Build history of the part. All positions in model axes, mm. Give positions to 0.01 mm unless a question says otherwise; leave off trailing zeros. Order: outer loops, then holes, each group sorted by start corner. A loop starts at its lowest first (then second) coordinate and runs counter-clockwise, first axis right, second up. Notation, with made-up numbers: (-15.75, -29.5) - (-4.75, -29.5) arc R22 ccw to (-4.75, -16.5) - close; hole circle Ø9 at (-6.5, 84.5). An arc over 180 degrees is marked (long way). Use a Markdown table: item, result.
from build123d import *

# Parameters (mm, degrees)
SKETCH2_W           = 30
SKETCH2_H           = 165
BOSS_EXTRUDE1_DEPTH = 8
SKETCH3_R           = 2.75
CUT_EXTRUDE1_DEPTH  = 8
SKETCH4_R           = 5
CUT_EXTRUDE2_DEPTH  = 4.2
SKETCH5_R           = 2.5
CUT_EXTRUDE3_DEPTH  = 41.2


with BuildPart() as part:
    # Sketch2 → Boss-Extrude1 (new body)
    with BuildSketch(Plane(origin=(0, 0, 0), x_dir=(1, 0, 0), z_dir=(0, 1, 0))):
        Rectangle(SKETCH2_W, SKETCH2_H)
    extrude(amount=BOSS_EXTRUDE1_DEPTH)

    # Sketch3 → Cut-Extrude1 (cut)
    with BuildSketch(Plane(origin=(0, 8, 0), x_dir=(1, 0, 0), z_dir=(0, 1, 0))):
        with Locations((0, -76.5)):
            Circle(SKETCH3_R)
        with Locations((0, 76.5)):
            Circle(SKETCH3_R)
    extrude(amount=-CUT_EXTRUDE1_DEPTH, mode=Mode.SUBTRACT)

    # Sketch4 → Cut-Extrude2 (cut)
    with BuildSketch(Plane(origin=(0, 8, 0), x_dir=(1, 0, 0), z_dir=(0, 1, 0))):
        with Locations((0, 76.5)):
            Circle(SKETCH4_R)
        with Locations((0, -76.5)):
            Circle(SKETCH4_R)
    extrude(amount=-CUT_EXTRUDE2_DEPTH, mode=Mode.SUBTRACT)

    # Sketch5 → Cut-Extrude3 (cut)
    with BuildSketch(Plane(origin=(0, 8, 0), x_dir=(1, 0, 0), z_dir=(0, 1, 0))):
        with Locations((-10, 76.5)):
            Circle(SKETCH5_R)
        with Locations((10, 76.5)):
            Circle(SKETCH5_R)
        with Locations((-10, -76.5)):
            Circle(SKETCH5_R)
        with Locations((10, -76.5)):
            Circle(SKETCH5_R)
    extrude(amount=-CUT_EXTRUDE3_DEPTH, mode=Mode.SUBTRACT)


solid = part.part
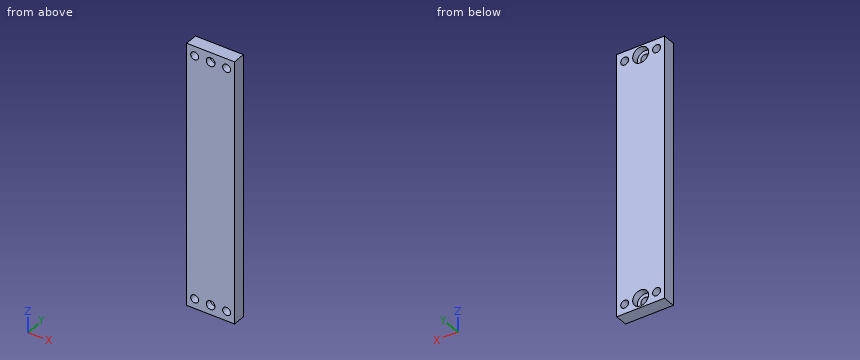
1) Wall check: line 1 (Z direction, x = 0, y = 5.6); line 2 (X direction, y = 3.5, z = 76.5); line 3 (Z direction, x = -10, y = 6.25). Give the ranges that are in metal, low to high. Write a range as from..to.
Computed:
| item | result |
|---|---|
| line 1 | z = -82.5..-81.5, -71.5..71.5, 81.5..82.5 |
| line 2 | x = -15..-12.5, -7.5..-2.75, 2.75..7.5, 12.5..15 |
| line 3 | z = -82.5..-79, -74..74, 79..82.5 |
2) Slice it at C-C (y = 6.5). Write the cut outline in (x, z), and give its area (3 significant figures).
Computed:
| item | result |
|---|---|
| outline | (-15, -82.5) - (15, -82.5) - (15, 82.5) - (-15, 82.5) - close; hole circle Ø5 at (-10, -76.5); hole circle Ø5 at (-10, 76.5); hole circle Ø10 at (0, -76.5); hole circle Ø10 at (0, 76.5); hole circle Ø5 at (10, -76.5); hole circle Ø5 at (10, 76.5) |
| area | 4,710 mm² |
3) Slice it at D-D (x = -10). Write the cut outline in (y, z).
Computed:
| item | result |
|---|---|
| outline | (0, -82.5) - (8, -82.5) - (8, -79) - (0, -79) - close; (0, -74) - (8, -74) - (8, 74) - (0, 74) - close; (0, 79) - (8, 79) - (8, 82.5) - (0, 82.5) - close |
4) Slice it at B-B (x = 0). Write the cut outline in (y, z), and give its area (3 significant figures).
Computed:
| item | result |
|---|---|
| outline | (0, -82.5) - (8, -82.5) - (8, -81.5) - (3.8, -81.5) - (3.8, -79.25) - (0, -79.25) - close; (0, -73.75) - (3.8, -73.75) - (3.8, -71.5) - (8, -71.5) - (8, 71.5) - (3.8, 71.5) - (3.8, 73.75) - (0, 73.75) - close; (0, 79.25) - (3.8, 79.25) - (3.8, 81.5) - (8, 81.5) - (8, 82.5) - (0, 82.5) - close |
| area | 1,190 mm² |
5) Slice it at A-A (z = -76.5). Write the cut outline in (x, y), and give its area (3 significant figures).
Computed:
| item | result |
|---|---|
| outline | (-15, 0) - (-12.5, 0) - (-12.5, 8) - (-15, 8) - close; (-7.5, 0) - (-2.75, 0) - (-2.75, 3.8) - (-5, 3.8) - (-5, 8) - (-7.5, 8) - close; (2.75, 0) - (7.5, 0) - (7.5, 8) - (5, 8) - (5, 3.8) - (2.75, 3.8) - close; (12.5, 0) - (15, 0) - (15, 8) - (12.5, 8) - close |
| area | 97.1 mm² |
